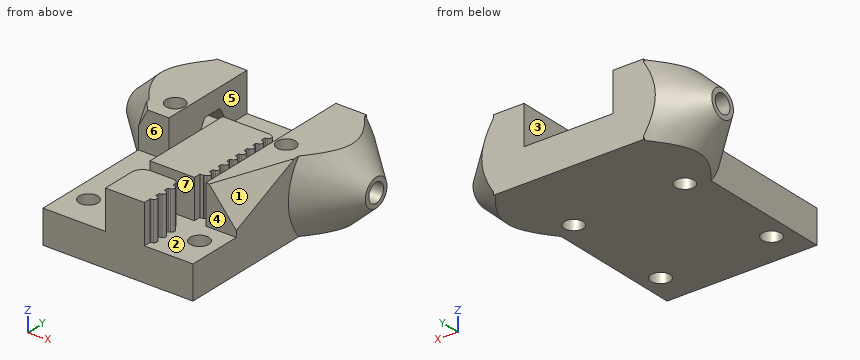
```python
from build123d import *

# Parameters (mm, degrees)
SKETCH064_R          = 1.7
PAD017_DEPTH         = 13
POCKET034_DEPTH      = 7
POCKET035_DEPTH      = 8
POCKET036_DEPTH      = 8
SKETCH069_R          = 2.5
SKETCH070_R          = 10
SKETCH072_R          = 10
SKETCH071_R          = 2.5
SKETCH066_R          = 1.7
POCKET037_DEPTH      = 21.5010001
POCKET037_DEPTH_BACK = 21.5010001
SKETCH073_W          = 57.890867
SKETCH073_H          = 28.005435
SKETCH073_W_2        = 40
SKETCH073_H_2        = 13
POCKET038_DEPTH      = 21.5010001
POCKET038_DEPTH_BACK = 21.5010001
SKETCH074_W          = 10.751613
SKETCH074_H          = 15.361299
POCKET039_DEPTH      = 5
SKETCH075_W          = 5.428132
SKETCH075_H          = 4.529939
POCKET040_DEPTH      = 5
FILLET012_R          = 2
FILLET013_R          = 1


with BuildPart() as part:
    # Sketch064 → Pad017 (new body)
    with BuildSketch(Plane.XY):
        Polygon((-13.5, -16), (13.5, -16), (13.5, 6), (13.5, 24), (-13.5, 24), (-13.5, 6), align=None)
        with Locations((10, 10)):
            Circle(SKETCH064_R, mode=Mode.SUBTRACT)
        with Locations((-10, 10)):
            Circle(SKETCH064_R, mode=Mode.SUBTRACT)
        with Locations((-10, -10)):
            Circle(SKETCH064_R, mode=Mode.SUBTRACT)
        with Locations((10, -10)):
            Circle(SKETCH064_R, mode=Mode.SUBTRACT)
    extrude(amount=PAD017_DEPTH)

    # Sketch065 → Pocket034 (cut)
    with BuildSketch(Plane.XY.offset(13)):
        with BuildLine():
            Line((-2.25, -16), (-2.25, -8))
            Line((-2.25, -8), (4.25, -8))
            Line((4.25, -8), (4.75, -8))
            Line((4.75, -8), (4.75, -9.2530602323))
            ThreePointArc((4.75, -9.2530602323), (4.7888446964, -9.3567216153), (4.8862469586, -9.4093276235))
            ThreePointArc((5.1882022472, -9.5011261235), (5.0408688943, -9.4432396073), (4.8862469586, -9.4093276235))
            ThreePointArc((5.1882022472, -10.4988789324), (5.5, -10.0000025279), (5.1882022472, -9.5011261235))
            ThreePointArc((4.8804347826, -10.5914594193), (5.038062154, -10.5576142423), (5.1882022472, -10.4988789324))
            ThreePointArc((4.8804347826, -10.5914594193), (4.7872285883, -10.641270882), (4.75, -10.740177953))
            Line((4.75, -10.740177953), (4.75, -11.259822047))
            ThreePointArc((4.75, -11.259822047), (4.7872285883, -11.358729118), (4.8804347826, -11.4085405807))
            ThreePointArc((5.1882022472, -11.5011210676), (5.038062154, -11.4423857578), (4.8804347826, -11.4085405807))
            ThreePointArc((5.1882022472, -12.4988738766), (5.5, -11.9999974721), (5.1882022472, -11.5011210676))
            ThreePointArc((4.8804347826, -12.5914543635), (5.038062154, -12.5576091865), (5.1882022472, -12.4988738766))
            ThreePointArc((4.8804347826, -12.5914543635), (4.7872285883, -12.6412658262), (4.75, -12.7401728972))
            Line((4.75, -12.7401728972), (4.75, -13.259822047))
            ThreePointArc((4.75, -13.259822047), (4.7872285883, -13.358729118), (4.8804347826, -13.4085405807))
            ThreePointArc((5.1882022472, -13.5011210676), (5.038062154, -13.4423857578), (4.8804347826, -13.4085405807))
            ThreePointArc((5.1882022472, -14.4988738766), (5.5, -13.9999974721), (5.1882022472, -13.5011210676))
            ThreePointArc((4.8804347826, -14.5914543635), (5.038062154, -14.5576091865), (5.1882022472, -14.4988738766))
            ThreePointArc((4.8804347826, -14.5914543635), (4.7872285871, -14.6412658275), (4.75, -14.7401729006))
            Line((4.75, -14.7401729006), (4.75, -16))
            Line((4.75, -16), (13.5, -16))
            Line((13.5, -16), (13.5, -6))
            Line((13.5, -6), (8, -6))
            Line((8, -6), (8, 1))
            Line((8, 24), (8, 1))
            Line((8, 24), (-8, 24))
            Line((-8, 24), (-8, 6))
            Line((-8, 6), (-13.5, 6))
            Line((-13.5, 6), (-13.5, -16))
            Line((-13.5, -16), (-2.25, -16))
        make_face()
        with BuildLine():
            Line((-2.25, 11), (5.75, 11))
            Line((6.38, 11), (5.75, 11))
            ThreePointArc((6.38, 11), (6.4172285895, 10.9010929313), (6.5104347826, 10.8512814699))
            ThreePointArc((6.8182022472, 10.758700983), (6.668062154, 10.8174362929), (6.5104347826, 10.8512814699))
            ThreePointArc((6.8182022472, 9.760948174), (7.13, 10.2598245785), (6.8182022472, 10.758700983))
            ThreePointArc((6.5104347826, 9.6683676871), (6.668062154, 9.7022128642), (6.8182022472, 9.760948174))
            ThreePointArc((6.5104347826, 9.6683676871), (6.4172285883, 9.6185562244), (6.38, 9.5196491534))
            Line((6.38, 9.5196491534), (6.38, 9.0000000036))
            ThreePointArc((6.38, 9.0000000036), (6.4172285883, 8.9010929326), (6.5104347826, 8.8512814699))
            ThreePointArc((6.8182022368, 8.7587009881), (6.6680621484, 8.8174362945), (6.5104347826, 8.8512814699))
            ThreePointArc((6.8182022368, 7.760948169), (7.13, 8.2598245785), (6.8182022368, 8.7587009881))
            ThreePointArc((6.5104347826, 7.6683676871), (6.6680621484, 7.7022128625), (6.8182022368, 7.760948169))
            ThreePointArc((6.5104347826, 7.6683676871), (6.4172285883, 7.6185562244), (6.38, 7.5196491534))
            Line((6.38, 7.5196491534), (6.38, 7.0000000036))
            ThreePointArc((6.38, 7.0000000036), (6.4172285883, 6.9010929326), (6.5104347826, 6.8512814699))
            ThreePointArc((6.8182022585, 6.7587009775), (6.66806216, 6.8174362911), (6.5104347826, 6.8512814699))
            ThreePointArc((6.8182022585, 5.7609481795), (7.13, 6.2598245785), (6.8182022585, 6.7587009775))
            ThreePointArc((6.5104347826, 5.6683676871), (6.66806216, 5.702212866), (6.8182022585, 5.7609481795))
            ThreePointArc((6.5104347826, 5.6683676871), (6.4172285883, 5.6185562244), (6.38, 5.5196491534))
            Line((6.38, 5.5196491534), (6.38, 5.0000000036))
            ThreePointArc((6.38, 5.0000000036), (6.4172285883, 4.9010929326), (6.5104347826, 4.8512814699))
            ThreePointArc((6.8182022472, 4.758700983), (6.668062154, 4.8174362929), (6.5104347826, 4.8512814699))
            ThreePointArc((6.8182022472, 3.760948174), (7.13, 4.2598245785), (6.8182022472, 4.758700983))
            ThreePointArc((6.5104347826, 3.6683676871), (6.668062154, 3.7022128642), (6.8182022472, 3.760948174))
            ThreePointArc((6.5104347826, 3.6683676871), (6.4172285883, 3.6185562244), (6.38, 3.5196491534))
            Line((6.38, 3.5196491534), (6.38, 3.0000000036))
            ThreePointArc((6.38, 3.0000000036), (6.4172285883, 2.9010929326), (6.5104347826, 2.8512814699))
            ThreePointArc((6.8182022472, 2.758700983), (6.668062154, 2.8174362929), (6.5104347826, 2.8512814699))
            ThreePointArc((6.8182022472, 1.760948174), (7.13, 2.2598245785), (6.8182022472, 2.758700983))
            ThreePointArc((6.5104347826, 1.6683676871), (6.668062154, 1.7022128642), (6.8182022472, 1.760948174))
            ThreePointArc((6.5104347826, 1.6683676871), (6.4172285883, 1.6185562244), (6.38, 1.5196491534))
            Line((6.38, 1.5196491534), (6.38, 1.0000000036))
            ThreePointArc((6.38, 1.0000000036), (6.4172285883, 0.9010929326), (6.5104347826, 0.8512814699))
            ThreePointArc((6.818202267, 0.7587009734), (6.6680621645, 0.8174362897), (6.5104347826, 0.8512814699))
            ThreePointArc((6.818202267, -0.2390518163), (7.13, 0.2598245785), (6.818202267, 0.7587009734))
            ThreePointArc((6.5104347826, -0.3316323129), (6.6680621645, -0.2977871326), (6.818202267, -0.2390518163))
            ThreePointArc((6.5104347826, -0.3316323129), (6.4172285883, -0.3814437756), (6.38, -0.4803508466))
            Line((6.38, -0.4803508466), (6.38, -0.9999999964))
            ThreePointArc((6.38, -0.9999999964), (6.4172285883, -1.0989070674), (6.5104347826, -1.1487185301))
            ThreePointArc((6.8182022472, -1.241299017), (6.668062154, -1.1825637071), (6.5104347826, -1.1487185301))
            ThreePointArc((6.8182022472, -2.239051826), (7.13, -1.7401754215), (6.8182022472, -1.241299017))
            ThreePointArc((6.5104347826, -2.3316323129), (6.668062154, -2.2977871358), (6.8182022472, -2.239051826))
            ThreePointArc((6.5104347826, -2.3316323129), (6.4172285883, -2.3814437756), (6.38, -2.4803508466))
            Line((6.38, -2.4803508466), (6.38, -2.9999999964))
            ThreePointArc((6.38, -2.9999999964), (6.4172285883, -3.0989070674), (6.5104347826, -3.1487185301))
            ThreePointArc((6.8182022472, -3.241299017), (6.668062154, -3.1825637071), (6.5104347826, -3.1487185301))
            ThreePointArc((6.8182022472, -4.239051826), (7.13, -3.7401754215), (6.8182022472, -3.241299017))
            ThreePointArc((6.5104347826, -4.3316323129), (6.668062154, -4.2977871358), (6.8182022472, -4.239051826))
            ThreePointArc((6.5104347826, -4.3316323129), (6.4172285873, -4.3814437767), (6.38, -4.4803508497))
            Line((5.75, -4.4803508497), (6.38, -4.4803508497))
            Line((5.75, -4.4803508497), (5.75, -5.7401754215))
            Line((5.75, -5.7401754215), (-2.25, -5.7401754215))
            Line((-2.25, 11), (-2.25, -5.7401754215))
        make_face(mode=Mode.SUBTRACT)
    extrude(amount=-POCKET034_DEPTH, mode=Mode.SUBTRACT)

    # Sketch067 → Pocket035 (cut)
    with BuildSketch(Plane.YZ.offset(4)):
        Polygon((19.5, 6.5), (17.75, 9.5310889133), (14.25, 9.5310889133), (12.5, 6.5), (14.25, 3.4689110868), (17.75, 3.4689110868), align=None)
    extrude(amount=POCKET035_DEPTH, mode=Mode.SUBTRACT)

    # Sketch068 → Pocket036 (cut)
    with BuildSketch(Plane.YZ.offset(-4)):
        Polygon((19.5, 6.5), (17.75, 9.5310889133), (14.25, 9.5310889133), (12.5, 6.5), (14.25, 3.4689110868), (17.75, 3.4689110868), align=None)
    extrude(amount=-POCKET036_DEPTH, mode=Mode.SUBTRACT)

    # Sketch069 → AdditiveLoft002 section 0
    with BuildSketch(Plane.YZ.offset(21.5)):
        with Locations((16, 6.5)):
            Circle(SKETCH069_R)
    # Sketch070 → AdditiveLoft002 section 1
    with BuildSketch(Plane.YZ.offset(13.5)):
        with Locations((16, 6.5)):
            Circle(SKETCH070_R)
    loft()

    # Sketch072 → AdditiveLoft003 section 0
    with BuildSketch(Plane.YZ.offset(-13.5)):
        with Locations((16, 6.5)):
            Circle(SKETCH072_R)
    # Sketch071 → AdditiveLoft003 section 1
    with BuildSketch(Plane.YZ.offset(-21.5)):
        with Locations((16, 6.5)):
            Circle(SKETCH071_R)
    loft()

    # Sketch066 → Pocket037 (cut, two sides)
    with BuildSketch(Plane.YZ) as pocket037_sk:
        with Locations((16, 6.5)):
            Circle(SKETCH066_R)
    extrude(amount=-POCKET037_DEPTH, mode=Mode.SUBTRACT)
    extrude(pocket037_sk.sketch, amount=POCKET037_DEPTH_BACK, mode=Mode.SUBTRACT)

    # Sketch073 → Pocket038 (cut, two sides)
    with BuildSketch(Plane.YZ) as pocket038_sk:
        with Locations((4.9093215, 6.8553455)):
            Rectangle(SKETCH073_W, SKETCH073_H)
        with Locations((4, 6.5)):
            Rectangle(SKETCH073_W_2, SKETCH073_H_2, mode=Mode.SUBTRACT)
    extrude(amount=-POCKET038_DEPTH, mode=Mode.SUBTRACT)
    extrude(pocket038_sk.sketch, amount=POCKET038_DEPTH_BACK, mode=Mode.SUBTRACT)

    # Sketch074 (on DatumPlane) → Pocket039 (cut)
    with BuildSketch(Plane(origin=(11.8478062442, -4.3122488143, 9.8505836052), x_dir=(0.5785325453, -0.210568626, -0.7880107536), z_dir=(0.7404878903, -0.2695155509, 0.6156614753))):
        with Locations((-0.9861515, 3.6505885)):
            Rectangle(SKETCH074_W, SKETCH074_H)
    extrude(amount=POCKET039_DEPTH, mode=Mode.SUBTRACT)

    # Sketch075 (on DatumPlane) → Pocket040 (cut)
    with BuildSketch(Plane(origin=(0, 0, 25), x_dir=(0.2777686245, 0.2484410627, 0.9279663947), z_dir=(-0.6924826787, -0.6177293717, 0.3726636058))):
        with Locations((-14.088813, 13.6448355)):
            Rectangle(SKETCH075_W, SKETCH075_H)
    extrude(amount=POCKET040_DEPTH, mode=Mode.SUBTRACT)

    # Fillet012
    fillet012_edges = [part.edges().sort_by_distance(p)[0] for p in [
        (-2.25, -8, 9.5),
    ]]
    fillet(fillet012_edges, radius=FILLET012_R)

    # Fillet013
    fillet013_edges = [part.edges().sort_by_distance(p)[0] for p in [
        (4.75, -8, 9.5),
    ]]
    fillet(fillet013_edges, radius=FILLET013_R)


solid = part.part
```
Geometry: final body of the model. Coordinates: model frame, mm. Face numbers are marked on the shaded views. A direction names the side the tool comes from. Round coordinates to 2 decimals unless told otherwise and drop trailing zeros. Loops run counter-clockwise (first coordinate to the right, second up) from the corner with the lowest first, then second, coordinate; pieces in that order, holes last. Notation, with made-up numbers: (87.5, -33) -> (118.5, -33) arc R6 cw to (118.5, -22) -> close; hole circle Ø2 at (-36.5, 86). An arc over 180 degrees is marked (long way). Use one line per item in the form item = value. Start each with the question number.
1) Line query: L1, parallel to X at y = -10, z = 3.95; L2, parallel to Y at x = 10, z = 3.4; L3, parallel to Y at x = 14.75, z = 6.5. Output: solid intervals per line, ascending.
2) First-contact query: P1, Ø4.5, axis at x = 2.5, z = 10, coming from the +Y side; P2, Ø1, axis at x = 7, y = 15, coming from the +Z side; P3, Ø1.9, axis at x = -0.5, y = 21.5, coming from the +Z side. Flat tips, straight axial feed; report the tip coordinate or a pass-through.
3) Section B-B on x = 0.5. Output: boundary loops of the cut face in (y, z).
4) Draft query along X for the marked faces 1, 2, 3 and 4. Return one class per face: released by +X, released by -X, zero draft, split by the parting line, or undercut.
5) Access query for the marked faces 5, 6 and 7. Directions: +Z, -Z, +X, -X, +Y, -Y. A direction counts if a zero-diameter tool reaches every point of the face in a straight line with its end or side. Return the directions, or none.
6) Section A-A on x = -10. Output: boundary loops of the cut face in (y, z), then the cut area to 3 significant figures.
7) Section D-D on y = -7.5. Output: boundary loops of the cut face in (x, z), then the cut area to 3 significant figures.
8) Section C-C on z = 10.5. Give the number of separate pieces and of enclosed holes in the cut face, then the cut area to 3 significant figures.
Response:
q1.L1 = -13.5 to -11.7, -8.3 to 8.3, 11.7 to 13.5
q1.L2 = -16 to -11.7, -8.3 to 8.3, 11.7 to 24
q1.L3 = 7.17 to 14.3, 17.7 to 24
q2.P1 = 11
q2.P2 = 3.47
q2.P3 = 6
q3.outline = (-16, 0) -> (24, 0) -> (24, 6) -> (17.62, 6) arc R1.7 cw to (14.38, 6) -> (11, 6) -> (11, 13) -> (-5.74, 13) -> (-5.74, 6) -> (-8, 6) -> (-8, 13) -> (-16, 13) -> close
q4.face_1 = released by +X
q4.face_2 = undercut
q4.face_3 = undercut
q4.face_4 = zero draft
q5.face_5 = +Z, +Y, -Y
q5.face_6 = +Z, -X, -Y
q5.face_7 = +Z, -X
q6.outline = (-16, 0) -> (-11.7, 0) -> (-11.7, 6) -> (-16, 6) -> close; (-8.3, 0) -> (8.3, 0) -> (8.3, 13) -> (6, 13) -> (6, 6) -> (-8.3, 6) -> close; (11.7, 0) -> (24, 0) -> (24, 13) -> (11.7, 13) -> close; hole (12.5, 6.5) -> (14.25, 3.47) -> (17.75, 3.47) -> (19.5, 6.5) -> (17.75, 9.53) -> (14.25, 9.53) -> close
q6.area = 270 mm^2
q7.outline = (-13.5, 0) -> (13.5, 0) -> (13.5, 6) -> (-13.5, 6) -> close
q7.area = 162 mm^2
q8.separate_pieces = 4
q8.enclosed_holes = 2
q8.area = 582 mm^2
